from build123d import *

# Parameters (mm, degrees)
F0_R     = 16
F0_R_2   = 7.5
F1_DEPTH = 130
F3_D     = 5.5
F3_DEPTH = 9
F3_TIP   = 1.6523667023
F4_D     = 5.5
F4_DEPTH = 9
F4_TIP   = 1.6523667023
F6_D     = 5.5
F6_DEPTH = 9
F6_TIP   = 1.6523667023
F7_D     = 5.5
F7_DEPTH = 9
F7_TIP   = 1.6523667023


with BuildPart() as f1:
    # F0 (on Top) → F1 (new body)
    with BuildSketch(Plane.XY):
        with Locations((0, -0.4519075282)):
            Circle(F0_R)
        with Locations((0, -0.4519075282)):
            Circle(F0_R_2, mode=Mode.SUBTRACT)
    extrude(amount=F1_DEPTH)

    # F3
    with Locations(Plane.XY.offset(130)):
        with Locations((0, 11.2980924718)):
            Hole(F3_D / 2, depth=F3_DEPTH)
            with Locations((0, 0, -(F3_DEPTH + F3_TIP / 2))):  # 118° drill point
                Cone(0, F3_D / 2, F3_TIP, mode=Mode.SUBTRACT)

    # F4
    with Locations(Plane.XY.offset(130)):
        with Locations((0, -12.2019075282)):
            Hole(F4_D / 2, depth=F4_DEPTH)
            with Locations((0, 0, -(F4_DEPTH + F4_TIP / 2))):  # 118° drill point
                Cone(0, F4_D / 2, F4_TIP, mode=Mode.SUBTRACT)

    # F6
    with Locations(Plane(origin=(0, 0, 0), x_dir=(1, 0, 0), z_dir=(0, 0, -1))):
        with Locations((0, -11.2980924718)):
            Hole(F6_D / 2, depth=F6_DEPTH)
            with Locations((0, 0, -(F6_DEPTH + F6_TIP / 2))):  # 118° drill point
                Cone(0, F6_D / 2, F6_TIP, mode=Mode.SUBTRACT)

    # F7
    with Locations(Plane(origin=(0, 0, 0), x_dir=(1, 0, 0), z_dir=(0, 0, -1))):
        with Locations((0, 12.2019075282)):
            Hole(F7_D / 2, depth=F7_DEPTH)
            with Locations((0, 0, -(F7_DEPTH + F7_TIP / 2))):  # 118° drill point
                Cone(0, F7_D / 2, F7_TIP, mode=Mode.SUBTRACT)


solid = f1.part
Source: CAD feature listing. Evaluate the final solid. Frame: model axes, mm. A direction names the side the tool comes from. Give positions to 0.01 mm unless a question says otherwise; leave off trailing zeros. Write each loop counter-clockwise with the first axis right and the second up, starting at its lowest first coordinate (ties: lowest second). Pieces come first, ordered by that corner, then holes. Notation, with made-up numbers: M 59.25,78 L 111.25,78 A22 ccw 111.25,99 Z; hole C 8.5,-25.75 d9. An arc over 180 degrees is marked long. Return JSON: item names as keys, results as strings. Group by question number.
1) Set-up query: faces 1 (the face through (0.6, -9.52, 4.56)), 2 (the face through (0.596, 8.613, 125.437)), 3 (the face through (7, -4, 0)). Return all of +Z, -Z, +X, -X, +Y, -Y with unobstructed straight access to the full face (end or side cutting, diameter ignored); none if empty.
2) Pull-direction query (Y, two-part tool) for faces 4 (the face through (-1.626, -7.774, 64.09)), 5 (the face through (15.261, 4.354, 64.09)), 6 (the face through (0.6, 13.98, 4.56)), 7 (the face through (7, -4, 130)); classes: pulls with the +Y half, pulls with the -Y half, needs draft (parallel to the pull), parting line crosses it, or undercut.
3) Material intervals for line 1 along Y through (x, z) = (0, 128); line 2 along Y through (x, z) = (-0.5, 67.5); line 3 along Y through (x, z) = (0, 39.5), sorted ascending. Write a range as [from, to].
4) Cut plane B-B, the plane x = -11. Output: boundary loops of the cut face in (y, z), plus the area to 3 significant figures.
5) Pin query (flat end, axial travel): P1, Ø4, axis at y = 2, z = 49, coming from the -X side; P2, Ø1, axis at y = 1.5, z = 81.5, coming from the +X side; P3, Ø1.5, axis at y = -3, z = 18, coming from the -X side. Return the tip coordinate at first contact, or that it passes through.
6) Cut plane A-A, the plane z = 63. Output: boundary loops of the cut face in (x, y).
Recorded:
{
 "1": {"face 1": "-Z", "face 2": "+Z", "face 3": "-Z, +X, -X, +Y, -Y"},
 "2": {"face 4": "undercut", "face 5": "parting line crosses it", "face 6": "undercut", "face 7": "needs draft"},
 "3": {"line 1": "y = [-16.45, -14.95], [-9.45, -7.95], [7.05, 8.55], [14.05, 15.55]", "line 2": "y = [-16.44, -7.94], [7.03, 15.54]", "line 3": "y = [-16.45, -7.95], [7.05, 15.55]"},
 "4": {"outline": "M -12.07,0 L 11.17,0 L 11.17,130 L -12.07,130 Z", "area": "3,020 mm²"},
 "5": {"P1": "stops at x = -15.99", "P2": "stops at x = 15.93", "P3": "stops at x = -15.9"},
 "6": {"outline": "C 0,-0.45 d32; hole C 0,-0.45 d15"}
}
